```python
from build123d import *
from build123d.topology import SkipClean

# Parameters (mm, degrees)
SKETCH1_R           = 28
SKETCH1_R_2         = 2
BOSS_EXTRUDE1_DEPTH = 39
SKETCH2_R           = 24
CUT_EXTRUDE1_DEPTH  = 27
CUT_EXTRUDE2_DEPTH  = 4
CUT_EXTRUDE4_DEPTH  = 56.578772926


with BuildPart() as part:
    # Sketch1 → Boss-Extrude1 (new body)
    with BuildSketch(Plane.XY):
        Circle(SKETCH1_R)
        Circle(SKETCH1_R_2, mode=Mode.SUBTRACT)
    extrude(amount=BOSS_EXTRUDE1_DEPTH)

    # Sketch2 → Cut-Extrude1 (cut)
    with BuildSketch(Plane(origin=(0, 0, 0), x_dir=(-1, 0, 0), z_dir=(0, 0, -1))):
        Circle(SKETCH2_R)
    extrude(amount=-CUT_EXTRUDE1_DEPTH, mode=Mode.SUBTRACT)

    # Sketch3 → Cut-Extrude2 (cut)
    with BuildSketch(Plane(origin=(0, 0, 27), x_dir=(-1, 0, 0), z_dir=(0, 0, -1))):
        Polygon((6, 0), (3, 5.196152423), (-3, 5.196152423), (-6, 0), (-3, -5.196152423), (3, -5.196152423), align=None)
    extrude(amount=-CUT_EXTRUDE2_DEPTH, mode=Mode.SUBTRACT)

    # Sketch5 → Cut-Extrude4 (cut, through all)
    with SkipClean():  # the faces are left unmerged after this step: merging them gives an invalid solid
        with BuildSketch(Plane.XY.offset(39)):
            with BuildLine():
                Line((-7, 22.956480566), (-2, 6.708203932))
                ThreePointArc((-2, 6.708203932), (0, 7), (2, 6.708203932))
                Line((2, 6.708203932), (7, 22.956480566))
                ThreePointArc((7, 22.956480566), (0, 24), (-7, 22.956480566))
            make_face()
            with BuildLine():
                Line((13.583670621, 19.785951897), (3.997705422, 5.746159706))
                ThreePointArc((3.997705422, 5.746159706), (5.472820377, 4.364428613), (6.491664629, 2.618833776))
                Line((6.491664629, 2.618833776), (22.312527847, 8.840311143))
                ThreePointArc((22.312527847, 8.840311143), (18.763955579, 14.963755245), (13.583670621, 19.785951897))
            make_face()
            with BuildLine():
                Line((23.938560207, 1.716197889), (6.985057122, 0.45714002))
                ThreePointArc((6.985057122, 0.45714002), (6.824495385, -1.557646538), (6.094973386, -3.442571629))
                Line((6.094973386, -3.442571629), (20.823267132, -11.932792881))
                ThreePointArc((20.823267132, -11.932792881), (23.398269892, -5.340502415), (23.938560207, 1.716197889))
            make_face()
            with BuildLine():
                Line((16.2672257, -17.645888133), (4.712518341, -5.176115424))
                ThreePointArc((4.712518341, -5.176115424), (3.037186174, -6.306782075), (1.108642869, -6.911650381))
                Line((1.108642869, -6.911650381), (3.65366155, -23.720260481))
                ThreePointArc((3.65366155, -23.720260481), (10.413209739, -21.62325283), (16.2672257, -17.645888133))
            make_face()
            with BuildLine():
                Line((-3.65366155, -23.720260481), (-1.108642869, -6.911650381))
                ThreePointArc((-1.108642869, -6.911650381), (-3.037186174, -6.306782075), (-4.712518341, -5.176115424))
                Line((-4.712518341, -5.176115424), (-16.2672257, -17.645888133))
                ThreePointArc((-16.2672257, -17.645888133), (-10.413209739, -21.62325283), (-3.65366155, -23.720260481))
            make_face()
            with BuildLine():
                Line((-20.823267132, -11.932792881), (-6.094973386, -3.442571629))
                ThreePointArc((-6.094973386, -3.442571629), (-6.824495385, -1.557646538), (-6.985057122, 0.45714002))
                Line((-6.985057122, 0.45714002), (-23.938560207, 1.716197889))
                ThreePointArc((-23.938560207, 1.716197889), (-23.398269892, -5.340502415), (-20.823267132, -11.932792881))
            make_face()
            with BuildLine():
                Line((-22.312527847, 8.840311143), (-6.491664629, 2.618833776))
                ThreePointArc((-6.491664629, 2.618833776), (-5.472820377, 4.364428613), (-3.997705422, 5.746159706))
                Line((-3.997705422, 5.746159706), (-13.583670621, 19.785951897))
                ThreePointArc((-13.583670621, 19.785951897), (-18.763955579, 14.963755245), (-22.312527847, 8.840311143))
            make_face()
        extrude(amount=-CUT_EXTRUDE4_DEPTH, mode=Mode.SUBTRACT)


solid = part.part
```
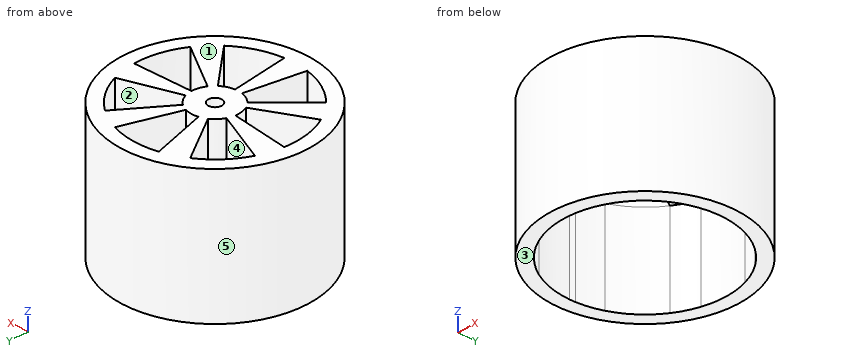
Input: part model. Units: mm. Frame: model coordinates. Face numbers are marked on the shaded views. A direction names the side the tool comes from. Round coordinates to 2 decimals unless told otherwise and drop trailing zeros. Loops run counter-clockwise (first coordinate to the right, second up) from the corner with the lowest first, then second, coordinate; pieces in that order, holes last. Notation, with made-up numbers: (-7.5, 84.25) -> (0.5, 84.25) arc R12 cw to (0.5, 106.25) -> close; hole circle Ø1 at (-29.75, 82.25). An arc over 180 degrees is marked (long way). Use one line per item in the form item = value. Start each with the question number.
Item 1: Material intervals for L1, parallel to Y at x = 0, z = 32.5; L2, parallel to Y at x = -0.5, z = 28.5; L3, parallel to X at y = -20, z = 32, sorted ascending. Write a range as from..to.
Item 2: Mould query, pull axis Y, two halves, no side actions, for the marked faces 3, 4 and 5. Classes: pulls with the +Y half, pulls with the -Y half, needs draft (parallel to the pull), parting line crosses it, or undercut.
Item 3: Set-up query: the marked faces 1 and 2. Return all of +Z, -Z, +X, -X, +Y, -Y with unobstructed straight access to the full face (end or side cutting, diameter ignored); none if empty.
Item 4: Contact query for flat-ended pins moving along their axis: pin 1 Ø1.5 at (x, z) = (9.5, 18.5) entering from +Y; pin 2 Ø1.2 at (x, z) = (-1.5, 28.5) entering from +Y; pin 3 Ø14 at (x, y) = (-3.5, -4) entering from -Z. Output: stop coordinate, or through.
Item 5: Section query C-C on y = 17.5. Return the cut outline in (x, z).
Item 6: Section query B-B on y = -13. Return the cut outline in (x, z).
Item 7: Section query D-D on z = 26. Return the cut outline in (x, y).
Item 8: Section query A-A on x = 0. Return the cut outline in (y, z).
Ans:
q1.L1 = -28..-2, 2..7, 24..28
q1.L2 = -28..-5.2, 5.2..6.98, 23.99..28
q1.L3 = -19.6..-13.27, -3.09..3.09, 13.27..19.6
q2.face_3 = needs draft
q2.face_4 = undercut
q2.face_5 = parting line crosses it
q3.face_1 = +Z, +X, -X, +Y, -Y
q3.face_2 = +Z, -Z
q4.pin_1 = 26.6
q4.pin_2 = 27.99
q4.pin_3 = 27
q5.outline = (-21.86, 0) -> (-16.42, 0) -> (-16.42, 39) -> (-21.86, 39) -> close; (-12.02, 27) -> (-5.32, 27) -> (-5.32, 39) -> (-12.02, 39) -> close; (5.32, 27) -> (12.02, 27) -> (12.02, 39) -> (5.32, 39) -> close; (16.42, 0) -> (21.86, 0) -> (21.86, 39) -> (16.42, 39) -> close
q6.outline = (-24.8, 0) -> (-20.17, 0) -> (-20.17, 27) -> (-11.96, 27) -> (-11.96, 39) -> (-24.8, 39) -> close; (-2.03, 27) -> (2.03, 27) -> (2.03, 39) -> (-2.03, 39) -> close; (11.96, 27) -> (20.17, 27) -> (20.17, 0) -> (24.8, 0) -> (24.8, 39) -> (11.96, 39) -> close
q7.outline = circle Ø56 at (0, 0); hole circle Ø48 at (0, 0)
q8.outline = (-28, 0) -> (-24, 0) -> (-24, 27) -> (-5.2, 27) -> (-5.2, 31) -> (-2, 31) -> (-2, 39) -> (-28, 39) -> close; (2, 31) -> (5.2, 31) -> (5.2, 27) -> (7, 27) -> (7, 39) -> (2, 39) -> close; (24, 0) -> (28, 0) -> (28, 39) -> (24, 39) -> close
